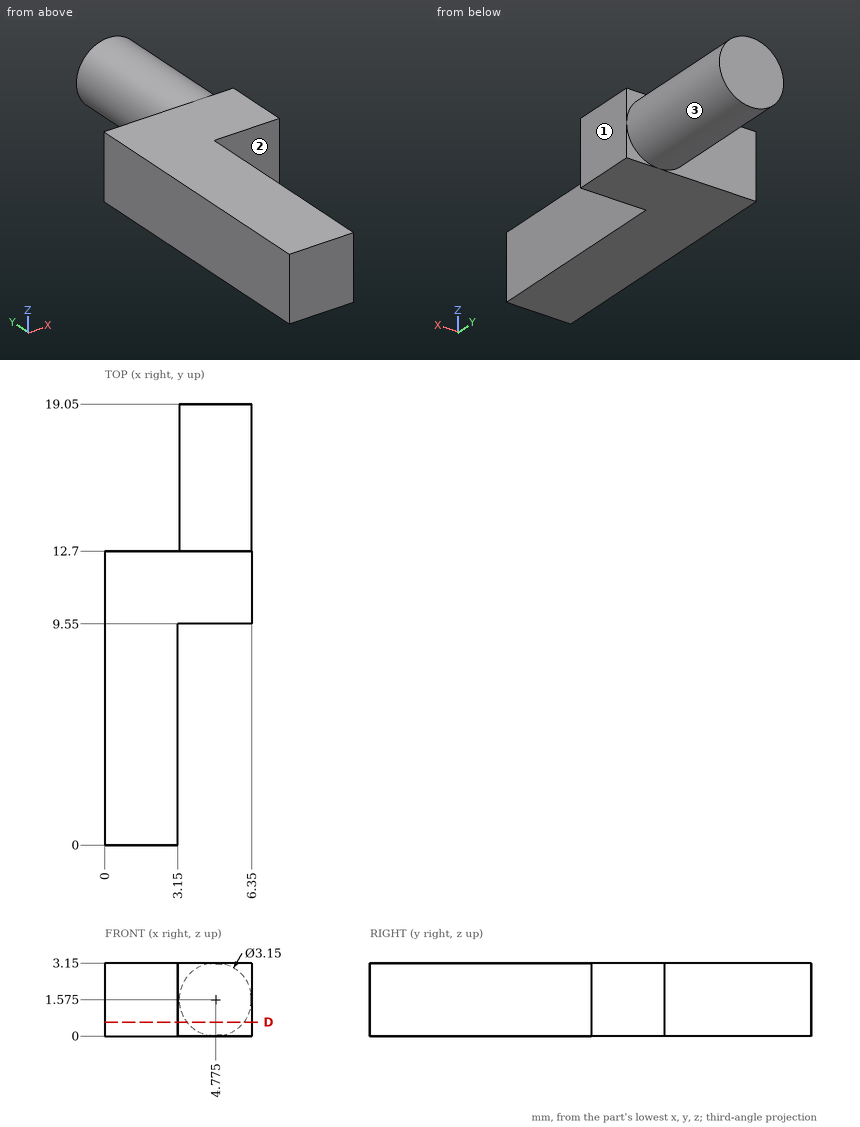
Here's the drawing with two shaded views (mm, measured from the low corner). I have some questions. A direction names the side the tool comes from. Coordinates: 2 decimals unless noted, no trailing zeros. Order: outer loops, then holes, each group sorted by start corner. A loop starts at its lowest first (then second) coordinate and runs counter-clockwise, first axis right, second up.
Item 1: If we section it at D-D, the plane z = 0.6: List the corners of the cut face in (x, y) for me.
Response values:
outline: (0, 0) - (3.15, 0) - (3.15, 9.55) - (6.35, 9.55) - (6.35, 12.7) - (6.01, 12.7) - (6.01, 19.05) - (3.54, 19.05) - (3.54, 12.7) - (0, 12.7) - close
Item 2: Which directions (+Z, -Z, +X, -X, +Y, -Y) give clear straight access to the entire face, cutting with the end or side of a thin tool? Please do the marked faces 1, 2 and 3.
Response values:
face 1: +Z, -Z, +X, +Y, -Y
face 2: +Z, -Z, +X, -Y
face 3: +Y
Item 3: I'm going to push flat-ended pins straight in: pin 1 Ø0.9 at (x, z) = (2, 2) entering from +Y; pin 2 Ø0.9 at (x, z) = (5.5, 2) entering from -Y. Where does each tip first touch, or does it pass through?
Response values:
pin 1: stops at y = 12.7
pin 2: stops at y = 9.55
Item 4: I need wall thicknesses on probe 1 along Y at (x, z) = (6.25, 0.85); probe 2 along X at (y, z) = (1, 0.55); probe 3 along Y at (x, z) = (3, 0.35). Which ranges of each line are inside material? Lowest first, please.
Response values:
probe 1: y = 9.55 to 12.7
probe 2: x = 0 to 3.15
probe 3: y = 0 to 12.7
